Autodesk Inventor part; units mm, degrees
ref_plane "YZ Plane" through (0, 0, 0) normal (1, 0, 0) x (0, 1, 0)
ref_plane "XZ Plane" through (0, 0, 0) normal (0, 1, 0) x (-1, 0, 0)
ref_plane "XY Plane" through (0, 0, 0) normal (0, 0, 1) x (1, 0, 0)
sketch "Sketch1" plane through (0, 0, 0) normal (0, 0, 1) x (1, 0, 0)
  line L0 (5, 2.8868) -> (5, -2.8868)
  line L1 (5, 2.8868) -> (0, 5.7735)
  line L2 (-5, 2.8868) -> (0, 5.7735)
  line L3 (0, -5.7735) -> (5, -2.8868)
  line L4 (-5, 2.8868) -> (-5, -2.8868)
  line L5 (-5, -2.8868) -> (0, -5.7735)
  point P0 (0, 0)
  point P1 (0, 0)
  point P2 (0, 0)
  point P3 (0, 0)
  point P4 (0, 0)
  dimension "d0" = 120
  dimension "d1" = 120
  dimension "d2" = 120
  dimension "d3" = 120
  dimension "d4" = 120
  dimension "d5" = 120
  dimension "d6" = 10
  dimension "d7" = 5
extrude "Extrusion1" add sketch "Sketch1" along normal blind 7
sketch "Sketch2" plane through (0, 0, 7) normal (0, 0, 1) x (1, 0, 0)
  point P0 (0, 0)
  point P1 (0, 0)
hole "Hole1" at (0, 0, 7) direction (0, 0, -1) diameter 4.134 end through all
properties part number "Nut-5" material "Steel, Mild"
Part model, mm, in its own coordinate system. Round coordinates to 2 decimals unless told otherwise and drop trailing zeros. Order: outer loops, then holes, each group sorted by start corner. A loop starts at its lowest first (then second) coordinate and runs counter-clockwise, first axis right, second up. Notation, with made-up numbers: M 11,61.5 L 63,61.5 A17 ccw 63,79.5 Z; hole C -8.75,38 d5. An arc over 180 degrees is marked long. Answer in a Markdown table with one row per item. Add a question column.
Q1. Cut at A-A on y = 0. Give the cut face in (x, z).
Q2. Cut at D-D on x = 3. Give the cut face in (y, z), and give its area (3 significant figures).
Q3. Cut at B-B on x = 1.75. Give the cut face in (y, z), and give its area (3 significant figures).
Q4. Wall check: L1, parallel to X at y = 0, z = 5; L2, parallel to Y at x = -0.75, z = 6.75; L3, parallel to X at y = 1.5, z = 2. Give the ranges that are in metal, low to high. Write a range as from..to.
Q5. Mould opens along X. For faces 1 (the face through (5, 0, 3)), 2 (the face through (-0.1, -2.5, 0)), 3 (the face through (-5, 0, 3)), 4 (the face through (1.26, 1.64, 3.45)) say: +X half, -X half, draft (parallel to the pull), parting line (faces both ways), or undercut.
Q6. Cut at C-C on z = 3.5. Give the cut face in (x, y), and give its area (3 significant figures).
Established:
| question | item | result |
|---|---|---|
| 1 | outline | M -5,0 L -2.07,0 L -2.07,7 L -5,7 Z; M 2.07,0 L 5,0 L 5,7 L 2.07,7 Z |
| 2 | outline | M -4.04,0 L 4.04,0 L 4.04,7 L -4.04,7 Z |
| 2 | area | 56.6 mm2 |
| 3 | outline | M -4.76,0 L -1.1,0 L -1.1,7 L -4.76,7 Z; M 1.1,0 L 4.76,0 L 4.76,7 L 1.1,7 Z |
| 3 | area | 51.3 mm2 |
| 4 | L1 | x = -5..-2.07, 2.07..5 |
| 4 | L2 | y = -5.34..-1.93, 1.93..5.34 |
| 4 | L3 | x = -5..-1.42, 1.42..5 |
| 5 | face 1 | +X half |
| 5 | face 2 | draft |
| 5 | face 3 | -X half |
| 5 | face 4 | undercut |
| 6 | outline | M -5,-2.89 L 0,-5.77 L 5,-2.89 L 5,2.89 L 0,5.77 L -5,2.89 Z; hole C 0,0 d4.13 |
| 6 | area | 73.2 mm2 |
